Answer from the drawing. Dimensions are ordinates in mm from the lowest x, y and z of the part. A direction names the side the tool comes from. Give positions to 0.01 mm unless a question says otherwise; leave off trailing zeros. Order: outer loops, then holes, each group sorted by start corner. A loop starts at its lowest first (then second) coordinate and runs counter-clockwise, first axis right, second up. Notation, with made-up numbers: (-25.75, -5.75) -> (4.25, -5.75) arc R27 cw to (4.25, 15.25) -> close; hole circle Ø6 at (66, 1.25). An arc over 180 degrees is marked (long way). Answer as a JSON object with one key per item and string values. Group by question number.
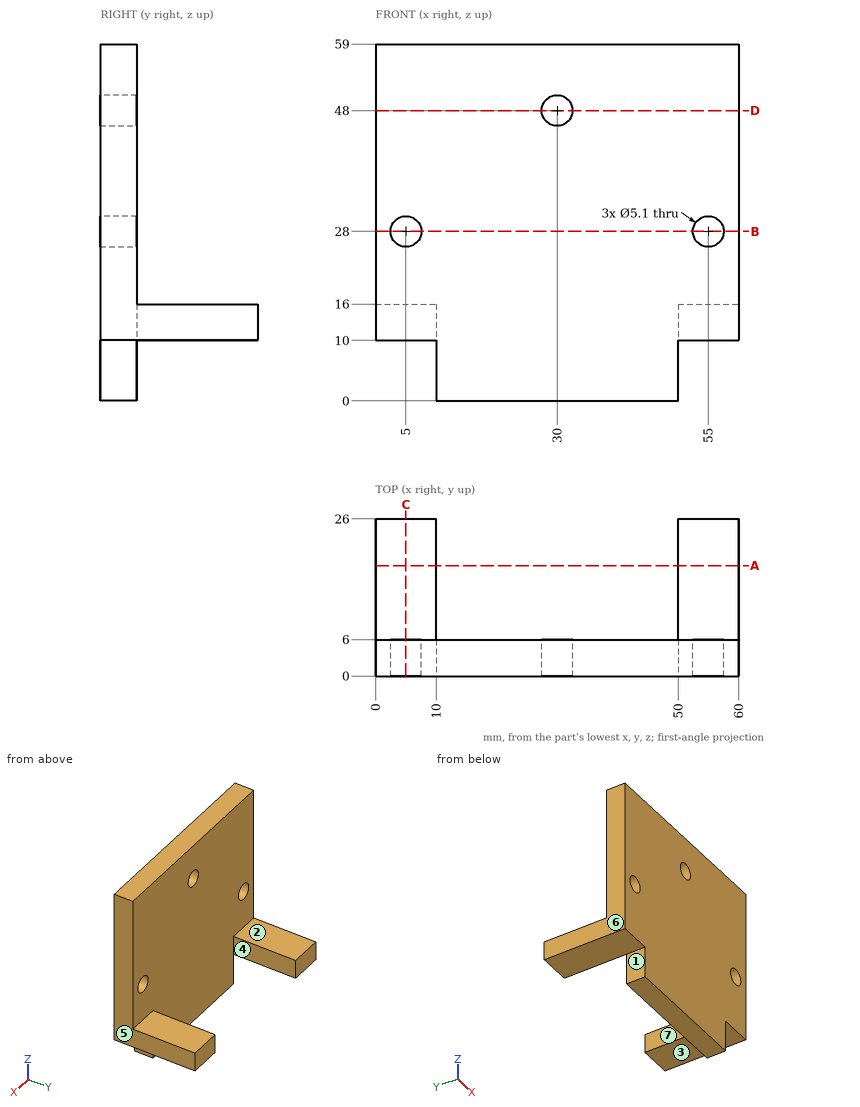
(1) A cutting plane is placed at D-D (z = 48). Determine the outline of the cut face in (x, y), and give its area (3 significant figures).
(2) Find the intervals of material crossed by line 1 along X through (y, z) = (19, 15); line 2 along X through (y, z) = (4.15, 28); line 3 along X through (y, z) = (2.25, 48), in increasing order. Write a range as [from, to].
(3) For a pull along X with two mould halves and no side action, classify the marked faces 5, 6 and 7 as +X half, -X half, draft (parallel to the pull), parting line (faces both ways), or undercut.
(4) A cutting plane is placed at C-C (x = 5). Determine the outline of the cut face in (y, z), and give its area (3 significant figures).
(5) A cutting plane is placed at B-B (z = 28). Determine the outline of the cut face in (x, y), and give its area (3 significant figures).
(6) Which of the six approach directions +Z, -Z, +X, -X, +Y, -Y give full straight-line access (tool end or side, diameter ignored) to the marked faces 1, 2, 3 and 4?
(7) A cutting plane is placed at A-A (y = 18.25). Determine the outline of the cut face in (x, z).
(8) Flat-ended cylindrical pins translate along their axes: pin 1 Ø3 at (x, y) = (55.5, 16.5) entering from +Z; pin 2 Ø4.5 at (x, z) = (30, 48) entering from +Y; pin 3 Ø12 at (x, z) = (41.5, 11) entering from +Y; pin 4 Ø5 at (x, y) = (5, 16) entering from -Z. Find the tip coordinate at first contact, or state that the pin passes through.
Check sheet entries:
{
 "1": {"outline": "(0, 0) -> (27.45, 0) -> (27.45, 6) -> (0, 6) -> close; (32.55, 0) -> (60, 0) -> (60, 6) -> (32.55, 6) -> close", "area": "329 mm2"},
 "2": {"line 1": "x = [0, 10], [50, 60]", "line 2": "x = [0, 2.45], [7.55, 52.45], [57.55, 60]", "line 3": "x = [0, 27.45], [32.55, 60]"},
 "3": {"face 5": "+X half", "face 6": "-X half", "face 7": "undercut"},
 "4": {"outline": "(0, 10) -> (26, 10) -> (26, 16) -> (6, 16) -> (6, 25.45) -> (0, 25.45) -> close; (0, 30.55) -> (6, 30.55) -> (6, 59) -> (0, 59) -> close", "area": "383 mm2"},
 "5": {"outline": "(0, 0) -> (2.45, 0) -> (2.45, 6) -> (0, 6) -> close; (7.55, 0) -> (52.45, 0) -> (52.45, 6) -> (7.55, 6) -> close; (57.55, 0) -> (60, 0) -> (60, 6) -> (57.55, 6) -> close", "area": "299 mm2"},
 "6": {"face 1": "-Z, -X, +Y, -Y", "face 2": "+Z, +X, -X, +Y", "face 3": "-Z, +X, +Y, -Y", "face 4": "+Z, -Z, +Y"},
 "7": {"outline": "(0, 10) -> (10, 10) -> (10, 16) -> (0, 16) -> close; (50, 10) -> (60, 10) -> (60, 16) -> (50, 16) -> close"},
 "8": {"pin 1": "stops at z = 16", "pin 2": "passes through", "pin 3": "stops at y = 6", "pin 4": "stops at z = 10"}
}
